Could you check a few things on this model? Use its own coordinates, in mm. A direction names the side the tool comes from. Give positions to 0.01 mm unless a question says otherwise; leave off trailing zeros. Loops run counter-clockwise (first coordinate to the right, second up) from the corner with the lowest first, then second, coordinate; pieces in that order, holes last. Notation, with made-up numbers: (-4.75, 81) -> (23.25, 81) arc R7 ccw to (23.25, 92) -> close; hole circle Ø7 at (45, 22). An arc over 180 degrees is marked (long way). Put each result on its own line as item: value.
```python
from build123d import *

# Parameters (mm, degrees)
SKETCH2_W             = 19.05
SKETCH2_H             = 19.05
BOSS_EXTRUDE1_DEPTH   = 48.05
BOSS_EXTRUDE1_2_DEPTH = 48.05
SKETCH3_W             = 142.49
SKETCH3_H             = 19.05
BOSS_EXTRUDE2_DEPTH   = 19.05


with BuildPart() as part:
    # Sketch2 → Boss-Extrude1 (new body)
    with BuildSketch(Plane(origin=(0, 0, 0), x_dir=(1, 0, 0), z_dir=(0, 1, 0))):
        with Locations((9.525, -9.525)):
            Rectangle(SKETCH2_W, SKETCH2_H)
    extrude(amount=BOSS_EXTRUDE1_DEPTH)



with BuildPart() as body_2:
    # Sketch2 → Boss-Extrude1 2 (new body)
    with BuildSketch(Plane(origin=(0, 0, 0), x_dir=(1, 0, 0), z_dir=(0, 1, 0))):
        with Locations((132.965, -9.525)):
            Rectangle(SKETCH2_W, SKETCH2_H)
    extrude(amount=BOSS_EXTRUDE1_2_DEPTH)


with BuildPart() as part_1:
    add(part.part)

    add(body_2.part)  # Boss-Extrude2 merges body 2
    # Sketch3 → Boss-Extrude2 (add)
    with BuildSketch(Plane(origin=(0, 48.05, 0), x_dir=(1, 0, 0), z_dir=(0, 1, 0))):
        with Locations((71.245, -9.525)):
            Rectangle(SKETCH3_W, SKETCH3_H)
    extrude(amount=BOSS_EXTRUDE2_DEPTH)


solid = part_1.part
```
1. Thinking about a two-plate mould opening in X: for faces 3 (the face through (0, 33, 10)), 4 (the face through (142.49, 33, 10)), 5 (the face through (71, 48.05, 9)), which applies, pulls with the +X half, pulls with the -X half, needs draft (parallel to the pull), parting line crosses it, or undercut?
Recorded:
face 3: pulls with the -X half
face 4: pulls with the +X half
face 5: undercut
2. For faces 1 (the face through (133, 0, 9)), 2 (the face through (123.44, 24, 10)), which set-ups out of +Z, -Z, +X, -X, +Y, -Y let a thin tool reach every point of the face, with its end or its side?
Recorded:
face 1: +Z, -Z, +X, -X, -Y
face 2: +Z, -Z, -Y
3. I'm going to push a flat-ended pin straight in: pin 1 (5.5 mm diameter, centred on x = 47.5, z = 13.5, fed in from -Y). Where does the tip first touch, or does it pass through?
Recorded:
pin 1: stops at y = 48.05
4. If we section it at B-B (z = 9.75): List the corners of the cut face in (x, y) for me.
Recorded:
outline: (0, 0) -> (19.05, 0) -> (19.05, 48.05) -> (123.44, 48.05) -> (123.44, 0) -> (142.49, 0) -> (142.49, 67.1) -> (0, 67.1) -> close
5. If we section it at C-C (x = 29.5): List the corners of the cut face in (y, z) for me.
Recorded:
outline: (48.05, 0) -> (67.1, 0) -> (67.1, 19.05) -> (48.05, 19.05) -> close
6. I need wall thicknesses on line 1 (X direction, y = 25, z = 3.75); line 2 (Y direction, x = 57, z = 10.5). Which ranges of each line are inside material? Lowest first, please.
Recorded:
line 1: x = 0 to 19.05, 123.44 to 142.49
line 2: y = 48.05 to 67.1
7. If we section it at A-A (y = 17): List the corners of the cut face in (x, z) for me, then the cut area to 3 significant figures.
Recorded:
outline: (0, 0) -> (19.05, 0) -> (19.05, 19.05) -> (0, 19.05) -> close; (123.44, 0) -> (142.49, 0) -> (142.49, 19.05) -> (123.44, 19.05) -> close
area: 726 mm^2
